Geometry: see drawing. Coordinates: mm, zero at the bounding-box minimum. Round coordinates to 2 decimals unless told otherwise and drop trailing zeros. Order: outer loops, then holes, each group sorted by start corner. A loop starts at its lowest first (then second) coordinate and runs counter-clockwise, first axis right, second up. Notation, with made-up numbers: (18, 43.25) -> (50, 43.25) arc R12 ccw to (50, 48.25) -> close; hole circle Ø11 at (58, 11). An arc over 180 degrees is marked (long way). Write item = value, one per line. Start each with the question number.
(1) Ray query, line 1 (X direction, y = 28.5, z = 54) (1 decimal); line 2 (Y direction, x = 37.5, z = 53) (1 decimal); line 3 (Y direction, x = 31, z = 11) (1 decimal). Return the intervals inside material, ascending.
(2) Cut plane C-C on x = 8.5. Return the cut outline in (y, z).
(3) Contact query for flat-ended pins moving along their axis: pin 1 Ø10 at (y, z) = (31.5, 46.5) entering from +X; pin 2 Ø2 at (x, z) = (7.5, 46) entering from -Y; pin 3 Ø1 at (y, z) = (6, 12.5) entering from -X (1 decimal). Output: stop coordinate, or through.
(4) Cut plane A-A on x = 20.32. Return the cut outline in (y, z).
(5) Cut plane B-B on y = 12.5. Return the cut outline in (x, z) (1 decimal).
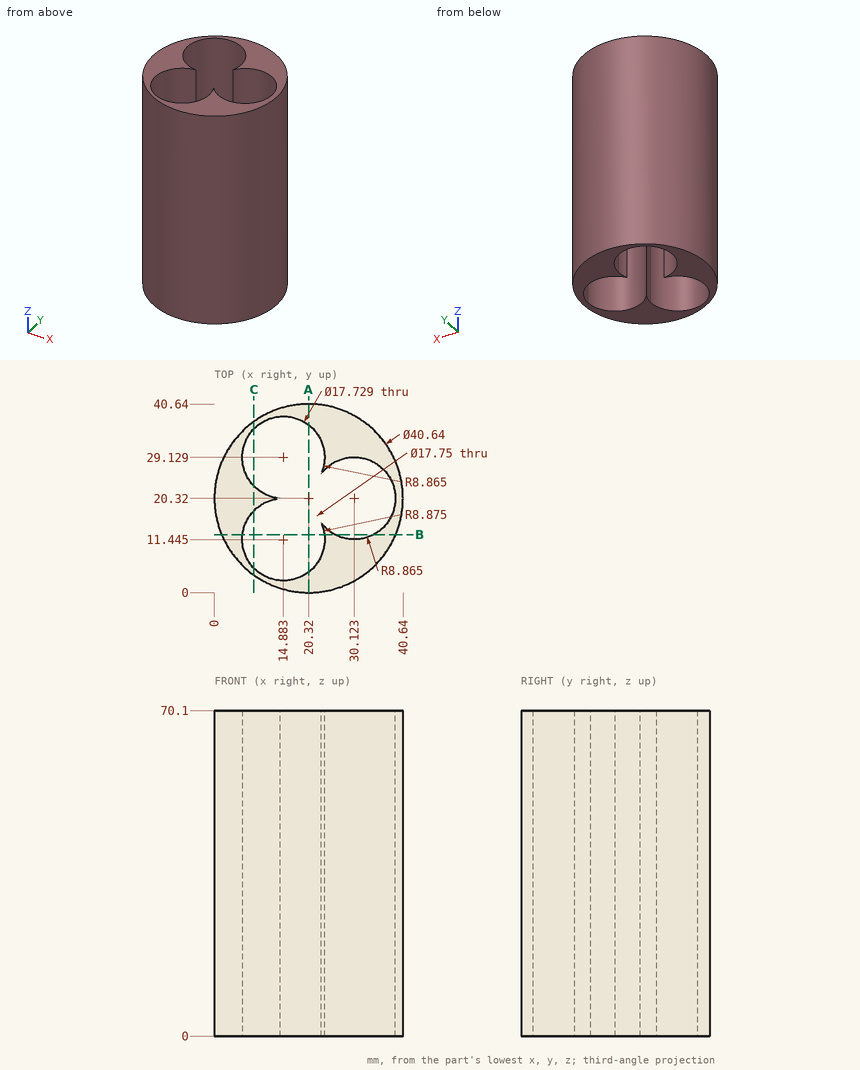
Evaluation:
q1.line_1 = 1.7 to 6, 23.7 to 26.7, 33.5 to 38.9
q1.line_2 = 9.5 to 15.4, 25.2 to 31.2
q1.line_3 = 3 to 11.5, 29.1 to 37.6
q2.outline = (3.79, 0) -> (5.28, 0) -> (5.28, 70.1) -> (3.79, 70.1) -> close; (17.61, 0) -> (22.98, 0) -> (22.98, 70.1) -> (17.61, 70.1) -> close; (35.28, 0) -> (36.85, 0) -> (36.85, 70.1) -> (35.28, 70.1) -> close
q3.pin_1 = 39.68
q3.pin_2 = 3.79
q3.pin_3 = 5.4
q4.outline = (0, 0) -> (4.43, 0) -> (4.43, 70.1) -> (0, 70.1) -> close; (36.13, 0) -> (40.64, 0) -> (40.64, 70.1) -> (36.13, 70.1) -> close
q5.outline = (1.6, 0) -> (6.1, 0) -> (6.1, 70.1) -> (1.6, 70.1) -> close; (23.7, 0) -> (25.9, 0) -> (25.9, 70.1) -> (23.7, 70.1) -> close; (34.3, 0) -> (39.1, 0) -> (39.1, 70.1) -> (34.3, 70.1) -> close
